Geometry: final body of the model. Coordinates: model frame, mm. A direction names the side the tool comes from. Give positions to 0.01 mm unless a question says otherwise; leave off trailing zeros. Write each loop counter-clockwise with the first axis right and the second up, starting at its lowest first coordinate (ties: lowest second). Pieces come first, ordered by that corner, then holes.
from build123d import *

# Parameters (mm, degrees)
BOSS_EXTRUDE1_DEPTH = 0.75
BOSS_EXTRUDE2_DEPTH = 3.75
BOSS_EXTRUDE3_DEPTH = 9.75
SKETCH1_5_W         = 0.75
SKETCH1_5_H         = 16
SKETCH1_5_H_2       = 8
BOSS_EXTRUDE4_DEPTH = 4.75
BOSS_EXTRUDE5_START = 9.75
SKETCH1_8_W         = 0.75
SKETCH1_8_H         = 8
BOSS_EXTRUDE5_DEPTH = 5


with BuildPart() as part:
    # Sketch1 → Boss-Extrude1 (new body)
    with BuildSketch(Plane(origin=(0, 0, 0), x_dir=(1, 0, 0), z_dir=(0, 1, 0))):
        with BuildLine():
            Line((0.75, 51.75), (80.25, 51.75))
            ThreePointArc((80.25, 51.75), (81.310660172, 51.310660172), (81.75, 50.25))
            Line((81.75, 50.25), (81.75, 0.75))
            ThreePointArc((81.75, 0.75), (81.310660172, -0.310660172), (80.25, -0.75))
            Line((80.25, -0.75), (0.75, -0.75))
            ThreePointArc((0.75, -0.75), (-0.310660172, -0.310660172), (-0.75, 0.75))
            Line((-0.75, 0.75), (-0.75, 50.25))
            ThreePointArc((-0.75, 50.25), (-0.310660172, 51.310660172), (0.75, 51.75))
        make_face()
    extrude(amount=BOSS_EXTRUDE1_DEPTH)

    # Sketch1_3 → Boss-Extrude2 (add)
    with BuildSketch(Plane(origin=(0, 0, 0), x_dir=(1, 0, 0), z_dir=(0, 1, 0))):
        with BuildLine():
            Line((10, 2), (0, 2))
            Line((0, 2), (0, 0.75))
            ThreePointArc((0, 0.75), (0.219669914, 0.219669914), (0.75, 0))
            Line((0.75, 0), (10, 0))
            Line((10, 0), (10, 2))
        make_face()
        with BuildLine():
            Line((0, 50.25), (0, 49))
            Line((0, 49), (10, 49))
            Line((10, 49), (10, 51))
            Line((10, 51), (0.75, 51))
            ThreePointArc((0.75, 51), (0.219669914, 50.780330086), (0, 50.25))
        make_face()
        with BuildLine():
            Line((80.25, 51), (71, 51))
            Line((71, 51), (71, 49))
            Line((71, 49), (81, 49))
            Line((81, 49), (81, 50.25))
            ThreePointArc((81, 50.25), (80.780330086, 50.780330086), (80.25, 51))
        make_face()
        with BuildLine():
            Line((71, 2), (71, 0))
            Line((71, 0), (80.25, 0))
            ThreePointArc((80.25, 0), (80.780330086, 0.219669914), (81, 0.75))
            Line((81, 0.75), (81, 2))
            Line((81, 2), (71, 2))
        make_face()
    extrude(amount=BOSS_EXTRUDE2_DEPTH)

    # Sketch1_4 → Boss-Extrude3 (add)
    with BuildSketch(Plane(origin=(0, 0, 0), x_dir=(1, 0, 0), z_dir=(0, 1, 0))):
        with BuildLine():
            Line((0, 2), (0, 21.5))
            Line((0, 21.5), (-0.75, 21.5))
            Line((-0.75, 21.5), (-0.75, 0.75))
            ThreePointArc((-0.75, 0.75), (-0.310660172, -0.310660172), (0.75, -0.75))
            Line((0.75, -0.75), (47, -0.75))
            Line((47, -0.75), (47, 0))
            Line((47, 0), (10, 0))
            Line((10, 0), (0.75, 0))
            ThreePointArc((0.75, 0), (0.219669914, 0.219669914), (0, 0.75))
            Line((0, 0.75), (0, 2))
        make_face()
        with BuildLine():
            Line((71, 0), (47, 0))
            Line((47, 0), (47, -0.75))
            Line((47, -0.75), (80.25, -0.75))
            ThreePointArc((80.25, -0.75), (81.310660172, -0.310660172), (81.75, 0.75))
            Line((81.75, 0.75), (81.75, 13.5))
            Line((81.75, 13.5), (81, 13.5))
            Line((81, 13.5), (81, 2))
            Line((81, 2), (81, 0.75))
            ThreePointArc((81, 0.75), (80.780330086, 0.219669914), (80.25, 0))
            Line((80.25, 0), (71, 0))
        make_face()
        with BuildLine():
            Line((47, 51.75), (47, 51))
            Line((47, 51), (71, 51))
            Line((71, 51), (80.25, 51))
            ThreePointArc((80.25, 51), (80.780330086, 50.780330086), (81, 50.25))
            Line((81, 50.25), (81, 49))
            Line((81, 49), (81, 21.5))
            Line((81, 21.5), (81.75, 21.5))
            Line((81.75, 21.5), (81.75, 50.25))
            ThreePointArc((81.75, 50.25), (81.310660172, 51.310660172), (80.25, 51.75))
            Line((80.25, 51.75), (47, 51.75))
        make_face()
        with BuildLine():
            Line((0, 37.5), (0, 49))
            Line((0, 49), (0, 50.25))
            ThreePointArc((0, 50.25), (0.219669914, 50.780330086), (0.75, 51))
            Line((0.75, 51), (10, 51))
            Line((10, 51), (47, 51))
            Line((47, 51), (47, 51.75))
            Line((47, 51.75), (0.75, 51.75))
            ThreePointArc((0.75, 51.75), (-0.310660172, 51.310660172), (-0.75, 50.25))
            Line((-0.75, 50.25), (-0.75, 37.5))
            Line((-0.75, 37.5), (0, 37.5))
        make_face()
    extrude(amount=BOSS_EXTRUDE3_DEPTH)

    # Sketch1_5 → Boss-Extrude4 (add)
    with BuildSketch(Plane(origin=(0, 0, 0), x_dir=(1, 0, 0), z_dir=(0, 1, 0))):
        with Locations((-0.375, 29.5)):
            Rectangle(SKETCH1_5_W, SKETCH1_5_H)
        with Locations((81.375, 17.5)):
            Rectangle(SKETCH1_5_W, SKETCH1_5_H_2)
    extrude(amount=BOSS_EXTRUDE4_DEPTH)

    # Sketch1_8 → Boss-Extrude5 (add)
    with BuildSketch(Plane(origin=(0, 0, 0), x_dir=(1, 0, 0), z_dir=(0, 1, 0)).offset(BOSS_EXTRUDE5_START)):
        with BuildLine():
            Line((71, 0), (47, 0))
            Line((47, 0), (47, -0.75))
            Line((47, -0.75), (80.25, -0.75))
            ThreePointArc((80.25, -0.75), (81.310660172, -0.310660172), (81.75, 0.75))
            Line((81.75, 0.75), (81.75, 13.5))
            Line((81.75, 13.5), (81, 13.5))
            Line((81, 13.5), (81, 2))
            Line((81, 2), (81, 0.75))
            ThreePointArc((81, 0.75), (80.780330086, 0.219669914), (80.25, 0))
            Line((80.25, 0), (71, 0))
        make_face()
        with Locations((81.375, 17.5)):
            Rectangle(SKETCH1_8_W, SKETCH1_8_H)
        with BuildLine():
            Line((47, 51.75), (47, 51))
            Line((47, 51), (71, 51))
            Line((71, 51), (80.25, 51))
            ThreePointArc((80.25, 51), (80.780330086, 50.780330086), (81, 50.25))
            Line((81, 50.25), (81, 49))
            Line((81, 49), (81, 21.5))
            Line((81, 21.5), (81.75, 21.5))
            Line((81.75, 21.5), (81.75, 50.25))
            ThreePointArc((81.75, 50.25), (81.310660172, 51.310660172), (80.25, 51.75))
            Line((80.25, 51.75), (47, 51.75))
        make_face()
    extrude(amount=BOSS_EXTRUDE5_DEPTH)


solid = part.part
Q1. Section B-B on x = 42.5. Output: boundary loops of the cut face in (y, z).
Filled sheet:
outline: (0, -51.75) - (9.75, -51.75) - (9.75, -51) - (0.75, -51) - (0.75, 0) - (9.75, 0) - (9.75, 0.75) - (0, 0.75) - close
Q2. Ray query, line 1 along X through (y, z) = (4.25, -42.5); line 2 along Z through (x, y) = (41, 5.5); line 3 along Y through (x, z) = (49.5, -16). Return the intervals inside material, ascending.
Filled sheet:
line 1: x = -0.75 to 0, 81 to 81.75
line 2: z = -51.75 to -51, 0 to 0.75
line 3: y = 0 to 0.75
Q3. Access query for faces 1 (the flat face through (-0.75, 4, -25)), 2 (the flat face through (5, 2, -2)). Directions: +Z, -Z, +X, -X, +Y, -Y. A direction counts if a zero-diameter tool reaches every point of the face in a straight line with its end or side. Return the directions, or none.
Filled sheet:
face 1: +Z, -Z, -X, +Y, -Y
face 2: +Y
Q4. Section D-D on z = -32. Output: boundary loops of the cut face in (x, y).
Filled sheet:
outline: (-0.75, 0) - (81.75, 0) - (81.75, 14.75) - (81, 14.75) - (81, 0.75) - (0, 0.75) - (0, 4.75) - (-0.75, 4.75) - close
Q5. Pull-direction query (X, two-part tool) for faces 3 (the flat face through (23, 9.75, 0.3)), 4 (the flat face through (41, 0.75, -26)), 5 (the cylindrical face through (81.32, 7.27, -51.3)); classes: released by +X, released by -X, zero draft, split by the parting line, or undercut.
Filled sheet:
face 3: zero draft
face 4: undercut
face 5: released by +X
Q6. Section C-C on y = 6.5. Output: boundary loops of the cut face in (x, z), plus the area to 3 significant figures.
Filled sheet:
outline: (-0.75, -50.25) arc R1.5 ccw to (0.75, -51.75) - (80.25, -51.75) arc R1.5 ccw to (81.75, -50.25) - (81.75, -21.5) - (81, -21.5) - (81, -50.25) arc R0.75 cw to (80.25, -51) - (0.75, -51) arc R0.75 cw to (0, -50.25) - (0, -37.5) - (-0.75, -37.5) - close; (-0.75, -21.5) - (0, -21.5) - (0, -0.75) arc R0.75 cw to (0.75, 0) - (80.25, 0) arc R0.75 cw to (81, -0.75) - (81, -13.5) - (81.75, -13.5) - (81.75, -0.75) arc R1.5 ccw to (80.25, 0.75) - (0.75, 0.75) arc R1.5 ccw to (-0.75, -0.75) - close
area: 181 mm2
Q7. Section A-A on y = 2.5. Output: boundary loops of the cut face in (x, z), plus the area to 3 significant figures.
Filled sheet:
outline: (-0.75, -50.25) arc R1.5 ccw to (0.75, -51.75) - (80.25, -51.75) arc R1.5 ccw to (81.75, -50.25) - (81.75, -0.75) arc R1.5 ccw to (80.25, 0.75) - (0.75, 0.75) arc R1.5 ccw to (-0.75, -0.75) - close; hole (0, -49) - (10, -49) - (10, -51) - (71, -51) - (71, -49) - (81, -49) - (81, -2) - (71, -2) - (71, 0) - (10, 0) - (10, -2) - (0, -2) - close
area: 278 mm2
Q8. Pin query (flat end, axial travel): P1, Ø1, axis at y = 10.5, z = -13, coming from the -X side; P2, Ø6, axis at x = 20, z = -44.5, coming from the -Y side; P3, Ø24.5, axis at x = 24, z = -6, coming from the +Y side; P4, Ø0.8, axis at x = -0.5, y = 6, coming from the +Z side. Return the tip coordinate at first contact, or that it passes through.
Filled sheet:
P1: stops at x = 81
P2: stops at y = 0
P3: stops at y = 9.75
P4: stops at z = 0.49
